For this review, take the finished solid that the model builds, in its own axes (mm). Give positions to 0.01 mm unless a question says otherwise; leave off trailing zeros. Answer as a JSON object with one key per item and string values. Group by question number.
```python
from build123d import *

# Parameters (mm, degrees)
SKETCH1_W           = 47.625
SKETCH1_H           = 47.625
BOSS_EXTRUDE1_DEPTH = 381
BOSS_EXTRUDE1_TAPER = 2.5
SKETCH2_R           = 3.429
CUT_EXTRUDE1_DEPTH  = 381
SKETCH5_W           = 47.625
SKETCH5_H           = 47.625
CUT_EXTRUDE4_DEPTH  = 190.5
SKETCH6_W           = 15.621
SKETCH6_H           = 15.621
SKETCH6_R           = 3.429
BOSS_EXTRUDE2_DEPTH = 6.35
BOSS_EXTRUDE2_TAPER = 30


with BuildPart() as part:
    # Sketch1 → Boss-Extrude1 (new body)
    with BuildSketch(Plane(origin=(0, 0, 0), x_dir=(1, 0, 0), z_dir=(0, 1, 0))):
        with Locations((23.8125, -23.8125)):
            Rectangle(SKETCH1_W, SKETCH1_H)
    extrude(amount=BOSS_EXTRUDE1_DEPTH, taper=BOSS_EXTRUDE1_TAPER)

    # Sketch2 → Cut-Extrude1 (cut)
    with BuildSketch(Plane.XZ):
        with Locations(Location((23.8125, 23.8125, 0), (0, 0, 270))):
            Circle(SKETCH2_R)
    extrude(amount=-CUT_EXTRUDE1_DEPTH, mode=Mode.SUBTRACT)

    # Sketch5 → Cut-Extrude4 (cut)
    with BuildSketch(Plane(origin=(0, 381, 0), x_dir=(1, 0, 0), z_dir=(0, 1, 0))):
        with Locations((23.8125, -23.8125)):
            Rectangle(SKETCH5_W, SKETCH5_H)
    extrude(amount=-CUT_EXTRUDE4_DEPTH, mode=Mode.SUBTRACT)

    # Sketch6 → Boss-Extrude2 (add)
    with BuildSketch(Plane(origin=(0, 190.5, 0), x_dir=(1, 0, 0), z_dir=(0, 1, 0))):
        with Locations((23.8125, -23.8125)):
            Rectangle(SKETCH6_W, SKETCH6_H)
        with Locations(Location((23.8125, -23.8125, 0), (0, 0, 90))):
            Circle(SKETCH6_R, mode=Mode.SUBTRACT)
    extrude(amount=BOSS_EXTRUDE2_DEPTH, taper=BOSS_EXTRUDE2_TAPER)


solid = part.part
```
Item 1: To check wall thickness, follow probe 1 along Y at (x, z) = (29, 36.5); probe 2 along Z at (x, y) = (45.5, 24.5); probe 3 along Z at (x, y) = (33, 101). State the ranges of each line that lie inside material, in increasing order.
Item 2: Draft analysis for pull direction X (two halves, no side actions). For faces 1 (the conical face through (27.408, 190.842, 24.285)), 2 (the flat face through (18, 0, 29)), 3 (the cylindrical face through (27.212, 93.916, 24.259)), state which applies: released by +X, released by -X, zero draft, split by the parting line, or undercut.
Item 3: Insertion check: P1, Ø6, axis at x = 11, y = 124, coming from the -Z side; P2, Ø3, axis at y = 138, z = 13, coming from the -X side; P3, Ø5, axis at x = 37.5, z = 26.5, coming from the +Y side. Each pin has a flat end and moves straight along its axis. Give the tip position at first contact, or say it passes through.
Result set:
{
 "1": {"probe 1": "y = 0 to 190.5", "probe 2": "z = 1.07 to 46.56", "probe 3": "z = 4.41 to 43.22"},
 "2": {"face 1": "undercut", "face 2": "zero draft", "face 3": "undercut"},
 "3": {"P1": "stops at z = 5.28", "P2": "stops at x = 5.96", "P3": "stops at y = 190.5"}
}
